Read the model definition and answer for the solid it produces. Units are mm, in the model's axes. Face numbers are marked on the shaded views. Give positions to 0.01 mm unless a question says otherwise; leave off trailing zeros. Order: outer loops, then holes, each group sorted by start corner. A loop starts at its lowest first (then second) coordinate and runs counter-clockwise, first axis right, second up. Notation, with made-up numbers: M 55.5,-40 L 77.5,-40 A18 cw 77.5,-23 Z; hole C 62,8 d11. An arc over 180 degrees is marked long. One line per item, written item: value.
from build123d import *

# Parameters (mm, degrees)
F0_R     = 8.575
F1_DEPTH = 26.5
F3_D     = 3.5
F4_D     = 3.5
F5_D     = 3.5


with BuildPart() as f1:
    # F0 (on Top) → F1 (new body)
    with BuildSketch(Plane.XY):
        Circle(F0_R)
    extrude(amount=F1_DEPTH)

    # F3 (through all)
    with Locations(Plane.XY.offset(26.5)):
        with Locations((0, 5.4)):
            Hole(F3_D / 2)

    # F4 (through all)
    with Locations(Plane.XY.offset(26.5)):
        with Locations((5.4, 0)):
            Hole(F4_D / 2)

    # F5 (through all)
    with Locations(Plane.XY.offset(26.5)):
        with Locations((-5.4, 0), (0, -5.4)):
            Hole(F5_D / 2)


solid = f1.part
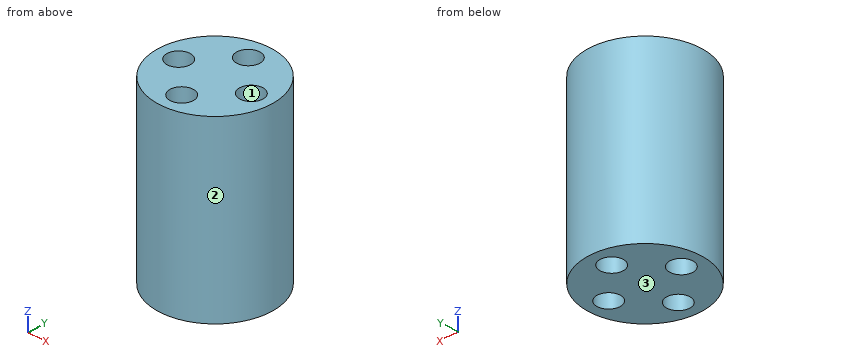
1) Each of these flat-tipped pins is pushed along its axis until it touches: pin 1 Ø5.5 at (x, y) = (-5.4, 0) entering from +Z; pin 2 Ø3 at (x, y) = (0, 5.4) entering from +Z; pin 3 Ø1.5 at (y, z) = (2, 17.5) entering from -X; pin 4 Ø4 at (y, z) = (5.5, 5.5) entering from -X. Where does it stop, or does it pass through?
Reported:
pin 1: stops at z = 26.5
pin 2: passes through
pin 3: stops at x = -8.48
pin 4: stops at x = -7.83
2) Find section D-D, the plane y = 5.4. Write down the section's boundary in (x, z).
Reported:
outline: M -6.66,0 L -1.75,0 L -1.75,26.5 L -6.66,26.5 Z; M 1.75,0 L 6.66,0 L 6.66,26.5 L 1.75,26.5 Z
3) Determine the mould class of the marked faces 1, 2 and 3 for opening direction X: +X half, -X half, draft (parallel to the pull), parting line (faces both ways), or undercut.
Reported:
face 1: undercut
face 2: parting line
face 3: draft
4) Find section B-B, the plane y = -0.5. Write down the section's boundary in (x, z), plus the area to 3 significant figures.
Reported:
outline: M -8.56,0 L -7.08,0 L -7.08,26.5 L -8.56,26.5 Z; M -3.72,0 L 3.72,0 L 3.72,26.5 L -3.72,26.5 Z; M 7.08,0 L 8.56,0 L 8.56,26.5 L 7.08,26.5 Z
area: 276 mm^2
5) Find section C-C, the plane z = 16.25. Write down the section's boundary in (x, y) (3 decimals).
Reported:
outline: C 0,0 d17.15; hole C -5.4,0 d3.5; hole C 0,-5.4 d3.5; hole C 0,5.4 d3.5; hole C 5.4,0 d3.5
6) Find section A-A, the plane x = 0. Write down the section's boundary in (y, z) (3 decimals).
Reported:
outline: M -8.575,0 L -7.15,0 L -7.15,26.5 L -8.575,26.5 Z; M -3.65,0 L 3.65,0 L 3.65,26.5 L -3.65,26.5 Z; M 7.15,0 L 8.575,0 L 8.575,26.5 L 7.15,26.5 Z
7) Consider probe 1 along Y at (x, z) = (0, 7.25) (3 decimals); probe 2 along Y at (x, z) = (-1, 24.5); probe 3 along X at (y, z) = (-0.5, 23.75). Determine where each line is inside the solid, lowest interval first.
Reported:
probe 1: y = -8.575 to -7.15, -3.65 to 3.65, 7.15 to 8.575
probe 2: y = -8.52 to -6.84, -3.96 to 3.96, 6.84 to 8.52
probe 3: x = -8.56 to -7.08, -3.72 to 3.72, 7.08 to 8.56
